The listing builds one solid part. Answer for the finished solid, in the listing's coordinates (mm). A direction names the side the tool comes from. Round coordinates to 2 decimals unless told otherwise and drop trailing zeros. Write each loop counter-clockwise with the first axis right and the second up, starting at its lowest first coordinate (ties: lowest second). Pieces come first, ordered by that corner, then holes.
Item 1: Find section D-D on x = -130.5. Give the vertices of the cut face in (y, z) (3 decimals), then the cut area to 3 significant figures.
Item 2: Find section B-B on x = 44.45. Give the vertices of the cut face in (y, z) (3 decimals), then the cut area to 3 significant figures.
Item 3: Find the intervals of material crossed by probe 1 along X at (y, z) = (5.3, -19.05); probe 2 along Z at (x, y) = (44.45, 4.3); probe 3 along Z at (x, y) = (-44, 4), in increasing order.
Item 4: Find section C-C on x = -28. Give the vertices of the cut face in (y, z) (3 decimals).
Item 5: Each of these flat-tipped pins is pushed along its axis until it touches: pin 1 (1.6 mm diameter, centred on x = -141.5, y = 4.5, fed in from -Z); pin 2 (9.5 mm diameter, centred on x = 92.075, z = -79.375, fed in from -Y) (3 decimals); pin 3 (1 mm diameter, centred on x = -156, y = 5.5, fed in from +Z); pin 4 (9.5 mm diameter, centred on x = -92.075, z = -79.375, fed in from +Y). Where does it stop, or does it pass through?
Item 6: For a pull along Z with two mould halves and no side action, classify faces 4 (the face through (1.6, -21, 118.1)), 5 (the face through (-114.3, -6, 113)), 6 (the face through (88.67, 4.74, -80.45)) as +Z half, -Z half, draft (parallel to the pull), parting line (faces both ways), or undercut.
Item 7: A tool of negligible diameter and unlimited length cuts with its end or side. For faces 1 (the face through (114.3, -6, -113)), 2 (the face through (-2, 3.175, -2)), 3 (the face through (114.3, -6, 113)), from which of +Z, -Z, +X, -X, +Y, -Y can it reach the whole face along a straight path? Write none if from no direction.
Item 8: Find section A-A on z = 44.45. Give the vertices of the cut face in (x, y) (3 decimals).
```python
from build123d import *

# Parameters (mm, degrees)
SKETCH1_W                   = 355.6
SKETCH1_H                   = 215.9
BOSS_EXTRUDE1_DEPTH         = 6.35
CONVERT_SOLID1_OUTLINE_W    = 355.6
CONVERT_SOLID1_OUTLINE_H    = 215.9
CONVERT_SOLID1_DEPTH        = 3.175
F_1_4_CLEARANCE_HOLE1_D     = 7.14248
F_1_4_START                 = 3.175
F_1_4_CLEARANCE_SLOT1_DEPTH = 3.175
EDGE_FLANGE2_DEPTH          = 228.6
EDGE_FLANGE2_BEND_DEPTH     = 228.6
FILLET1_R                   = 12.7
FILLET2_R                   = 25.4


# Read off the part's stored shape, not the designer's step: Convert-Solid1, 1/4 Clearance Slot1
# Sheet-metal steps are written as plain solids
with BuildPart() as part:
    # Sketch1 → Boss-Extrude1 (new body)
    with BuildSketch(Plane(origin=(0, 0, 0), x_dir=(1, 0, 0), z_dir=(0, 1, 0))):
        Rectangle(SKETCH1_W, SKETCH1_H)
    extrude(amount=BOSS_EXTRUDE1_DEPTH)

    # Convert-Solid1 outline → Convert-Solid1 (cut)
    with BuildSketch(Plane(origin=(0, 0, 0), x_dir=(1, 0, 0), z_dir=(0, 1, 0))):
        Rectangle(CONVERT_SOLID1_OUTLINE_W, CONVERT_SOLID1_OUTLINE_H)
    extrude(amount=CONVERT_SOLID1_DEPTH, mode=Mode.SUBTRACT)

    # 1/4 Clearance Hole1 (through all)
    with Locations(Plane(origin=(0, 6.35, 0), x_dir=(1, 0, 0), z_dir=(0, 1, 0))):
        with Locations((-92.075, 79.375), (-44.45, 19.05), (44.45, 19.05), (-44.45, -44.45), (44.45, -44.45), (92.075, 79.375), (155.575, 79.375), (155.575, -85.725)):
            Hole(F_1_4_CLEARANCE_HOLE1_D / 2)

    # 1/4 Clearance Slot1 outline → 1/4 Clearance Slot1 (cut)
    with BuildSketch(Plane(origin=(0, 0, 0), x_dir=(1, 0, 0), z_dir=(0, 1, 0)).offset(F_1_4_START)):
        with BuildLine():
            Line((-158.35376, -89.29624), (-152.79624, -89.29624))
            ThreePointArc((-152.79624, -89.29624), (-149.225, -85.725), (-152.79624, -82.15376))
            Line((-152.79624, -82.15376), (-158.35376, -82.15376))
            ThreePointArc((-158.35376, -82.15376), (-161.925, -85.725), (-158.35376, -89.29624))
        make_face()
        with BuildLine():
            Line((-158.35376, 75.80376), (-152.79624, 75.80376))
            ThreePointArc((-152.79624, 75.80376), (-149.225, 79.375), (-152.79624, 82.94624))
            Line((-152.79624, 82.94624), (-158.35376, 82.94624))
            ThreePointArc((-158.35376, 82.94624), (-161.925, 79.375), (-158.35376, 75.80376))
        make_face()
    extrude(amount=F_1_4_CLEARANCE_SLOT1_DEPTH, mode=Mode.SUBTRACT)

    # Edge-Flange2 section (across the edge) → Edge-Flange2 (add)
    with BuildSketch(Plane(origin=(-114.3, 3.175, -110.614141329), x_dir=(0, -0.17364817766693427, 0.9848077530122075), z_dir=(1, 0, 0))):
        with BuildLine():
            Line((-3.175, 2.664141329), (-3.175, 48.135858671))
            Line((-3.175, 48.135858671), (0, 48.135858671))
            Line((0, 48.135858671), (0, 2.664141329))
            ThreePointArc((0, 2.664141329), (0.742808893, 0.623290668), (2.623667036, -0.462623287))
            Line((2.623667036, -0.462623287), (2.072334072, -3.589387903))
            ThreePointArc((2.072334072, -3.589387903), (-1.689382214, -1.417559993), (-3.175, 2.664141329))
        make_face()
    extrude(amount=EDGE_FLANGE2_DEPTH)

    # Edge-Flange2 section 2 (across the edge) → Edge-Flange2 bend (add)
    with BuildSketch(Plane(origin=(114.3, 3.175, 110.614141329), x_dir=(0, -0.17364817766693427, -0.9848077530122075), z_dir=(-1, 0, 0))):
        with BuildLine():
            Line((-3.175, 2.664141329), (-3.175, 48.135858671))
            Line((-3.175, 48.135858671), (0, 48.135858671))
            Line((0, 48.135858671), (0, 2.664141329))
            ThreePointArc((0, 2.664141329), (0.742808893, 0.623290668), (2.623667036, -0.462623287))
            Line((2.623667036, -0.462623287), (2.072334072, -3.589387903))
            ThreePointArc((2.072334072, -3.589387903), (-1.689382214, -1.417559993), (-3.175, 2.664141329))
        make_face()
    extrude(amount=EDGE_FLANGE2_BEND_DEPTH)

    # Fillet1
    fillet1_edges = [part.edges().sort_by_distance(p)[0] for p in [
        (177.8, 4.7625, -107.95),
        (177.8, 4.7625, 107.95),
        (-177.8, 4.7625, 107.95),
        (-177.8, 4.7625, -107.95),
    ]]
    fillet(fillet1_edges, radius=FILLET1_R)

    # Fillet2
    fillet2_edges = [part.edges().sort_by_distance(p)[0] for p in [
        (-114.3, -43.953900335, -120.536227776),
        (114.3, -43.953900335, -120.536227776),
        (114.3, -43.953900335, 120.536227776),
        (-114.3, -43.953900335, 120.536227776),
    ]]
    fillet(fillet2_edges, radius=FILLET2_R)


solid = part.part
```
Check values:
1. outline: (3.175, -107.95) - (6.35, -107.95) - (6.35, 107.95) - (3.175, 107.95) - close
1. area: 685 mm2
2. outline: (-44.23, -118.973) - (-43.678, -122.1) - (1.103, -114.204) arc R6.35 ccw to (6.35, -107.95) - (6.35, -22.621) - (3.175, -22.621) - (3.175, -107.95) arc R3.175 cw to (0.551, -111.077) - close; (-44.23, 118.973) - (0.551, 111.077) arc R3.175 cw to (3.175, 107.95) - (3.175, 48.021) - (6.35, 48.021) - (6.35, 107.95) arc R6.35 ccw to (1.103, 114.204) - (-43.678, 122.1) - close; (3.175, -15.479) - (6.35, -15.479) - (6.35, 40.879) - (3.175, 40.879) - close
2. area: 971 mm2
3. probe 1: x = -177.8 to -48.02, -40.88 to 40.88, 48.02 to 177.8
3. probe 2: z = -112.62 to -22.62, -15.48 to 40.88, 48.02 to 112.62
3. probe 3: z = -112.88 to -22.59, -15.51 to 40.91, 47.99 to 112.88
4. outline: (-44.23, -118.973) - (-43.678, -122.1) - (1.103, -114.204) arc R6.35 ccw to (6.35, -107.95) - (6.35, 107.95) arc R6.35 ccw to (1.103, 114.204) - (-43.678, 122.1) - (-44.23, 118.973) - (0.551, 111.077) arc R3.175 cw to (3.175, 107.95) - (3.175, -107.95) arc R3.175 cw to (0.551, -111.077) - close
5. pin 1: stops at z = -107.95
5. pin 2: stops at y = 3.175
5. pin 3: stops at z = 107.95
5. pin 4: stops at y = 6.35
6. face 4: +Z half
6. face 5: draft
6. face 6: undercut
7. face 1: -Z, +X, +Y, -Y
7. face 2: +X, -X, -Y
7. face 3: +Z, +X, +Y, -Y
8. outline: (-177.8, 3.175) - (-48.021, 3.175) - (-48.021, 6.35) - (-177.8, 6.35) - close; (-40.879, 3.175) - (40.879, 3.175) - (40.879, 6.35) - (-40.879, 6.35) - close; (48.021, 3.175) - (177.8, 3.175) - (177.8, 6.35) - (48.021, 6.35) - close
